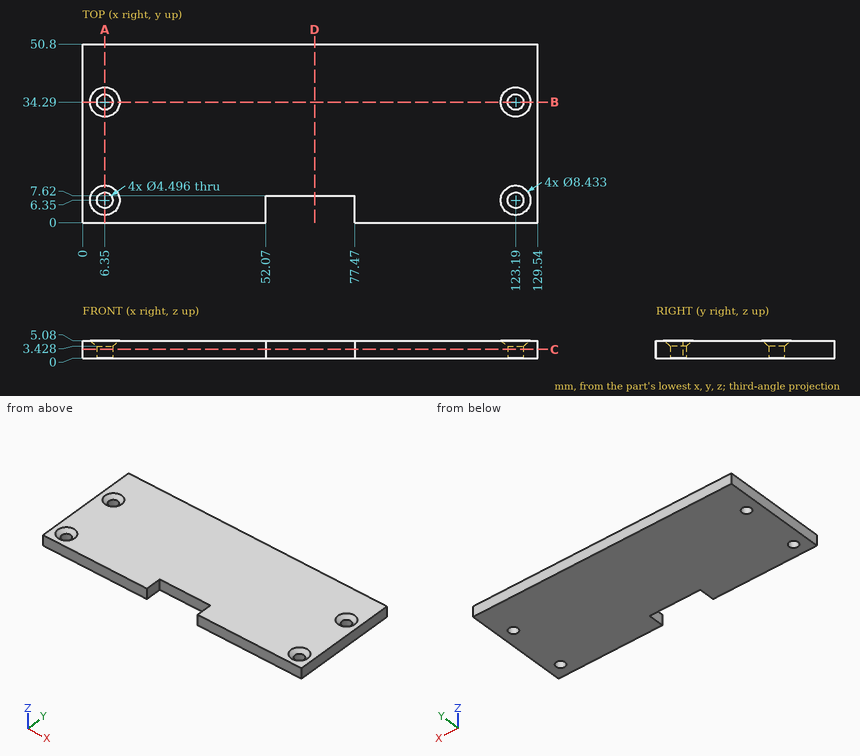
Verification items for this drawing (mm, ordinates from the low corner). Coordinates: 2 decimals unless noted, no trailing zeros. Order: outer loops, then holes, each group sorted by start corner. A loop starts at its lowest first (then second) coordinate and runs counter-clockwise, first axis right, second up.
Q1. Sectioned sample at B-B on y = 34.29. Record the cut outline in (x, z).
Reply:
outline: (0, 0) - (4.1, 0) - (4.1, 3.43) - (2.13, 5.08) - (0, 5.08) - close; (8.6, 0) - (120.94, 0) - (120.94, 3.43) - (118.97, 5.08) - (10.57, 5.08) - (8.6, 3.43) - close; (125.44, 0) - (129.54, 0) - (129.54, 5.08) - (127.41, 5.08) - (125.44, 3.43) - close
Q2. Sectioned sample at C-C on z = 2.55. Record the cut outline in (x, y).
Reply:
outline: (0, 0) - (52.07, 0) - (52.07, 7.62) - (77.47, 7.62) - (77.47, 0) - (129.54, 0) - (129.54, 50.8) - (0, 50.8) - close; hole circle Ø4.5 at (6.35, 6.35); hole circle Ø4.5 at (6.35, 34.29); hole circle Ø4.5 at (123.19, 6.35); hole circle Ø4.5 at (123.19, 34.29)
Q3. Thickness scan on probe 1 along X at (y, z) = (34.29, 2.65); probe 2 along X at (y, z) = (34.5, 3.2); probe 3 along Y at (x, z) = (6.35, 1.8). Record the ranges inside material, lowest first.
Reply:
probe 1: x = 0 to 4.1, 8.6 to 120.94, 125.44 to 129.54
probe 2: x = 0 to 4.11, 8.59 to 120.95, 125.43 to 129.54
probe 3: y = 0 to 4.1, 8.6 to 32.04, 36.54 to 50.8
Q4. Sectioned sample at D-D on x = 66. Record the cut outline in (y, z), and give its area (3 significant figures).
Reply:
outline: (7.62, 0) - (50.8, 0) - (50.8, 5.08) - (7.62, 5.08) - close
area: 219 mm2
Q5. Sectioned sample at A-A on x = 6.35. Record the cut outline in (y, z), and give its area (3 significant figures).
Reply:
outline: (0, 0) - (4.1, 0) - (4.1, 3.43) - (2.13, 5.08) - (0, 5.08) - close; (8.6, 0) - (32.04, 0) - (32.04, 3.43) - (30.07, 5.08) - (10.57, 5.08) - (8.6, 3.43) - close; (36.54, 0) - (50.8, 0) - (50.8, 5.08) - (38.51, 5.08) - (36.54, 3.43) - close
area: 206 mm2
